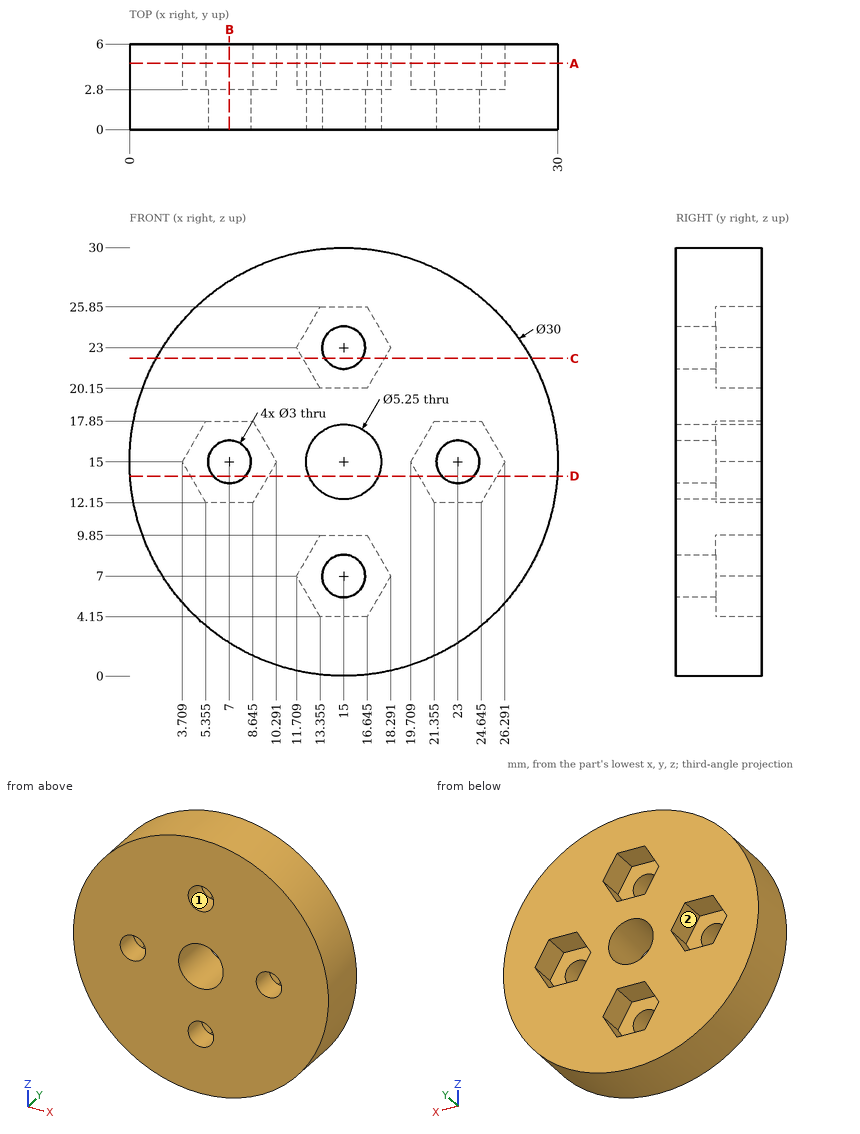
Source: three-view drawing plus pictorial views. Frame: mm from the lowest corner of the part. A direction names the side the tool comes from. Give positions to 0.01 mm unless a question says otherwise; leave off trailing zeros. Order: outer loops, then holes, each group sorted by start corner. A loop starts at its lowest first (then second) coordinate and runs counter-clockwise, first axis right, second up. Notation, with made-up numbers: M -30.5,26.25 L 25.5,26.25 A27 cw 25.5,47.25 Z; hole C 5,86 d5. An arc over 180 degrees is marked long. One line per question, with ' | ' between items. Start each with the question number.
1. First-contact query: pin 1 Ø1.6 at (x, y) = (7, 4) entering from -Z; pin 2 Ø5 at (x, z) = (15, 23) entering from +Y; pin 3 Ø2.5 at (x, y) = (23, 5) entering from -Z (1 decimal). Flat tips, straight axial feed; report the tip coordinate or a pass-through.
2. Material intervals for probe 1 along Z at (x, y) = (18, 4.4) (1 decimal); probe 2 along Z at (x, y) = (15.5, 2.85); probe 3 along X at (y, z) = (4, 14) (1 decimal), sorted ascending. Write a range as [from, to].
3. Access query for the marked faces 1 and 2. Directions: +Z, -Z, +X, -X, +Y, -Y. A direction counts if a zero-diameter tool reaches every point of the face in a straight line with its end or side. Return the directions, or none.
4. Section query C-C (z = 22.25). Return the cut outline in (x, y).
5. Section query A-A (y = 4.65). Count the separate pieces of the cut face and the enclosed holes in it.
6. Section query D-D (z = 14). Return the cut outline in (x, y), and give its area (3 significant figures).
7. Section query B-B (x = 7). Return the cut outline in (y, z), and give its area (3 significant figures).
Here are the results:
1) pin 1: z = 1.84 | pin 2: y = 2.8 | pin 3: z = 1.6
2) probe 1: [0.3, 6.5], [7.5, 22.5], [23.5, 29.7] | probe 2: [0.01, 4.15], [9.85, 12.42], [17.58, 20.15], [25.85, 29.99] | probe 3: [0, 4.3], [9.7, 12.6], [17.4, 20.3], [25.7, 30]
3) face 1: +Y, -Y | face 2: +Y
4) outline: M 1.87,0 L 13.7,0 L 13.7,2.8 L 12.14,2.8 L 12.14,6 L 1.87,6 Z; M 16.3,0 L 28.13,0 L 28.13,6 L 17.86,6 L 17.86,2.8 L 16.3,2.8 Z
5) separate pieces: 1 | enclosed holes: 5
6) outline: M 0.03,0 L 5.88,0 L 5.88,2.8 L 4.29,2.8 L 4.29,6 L 0.03,6 Z; M 8.12,0 L 12.57,0 L 12.57,6 L 9.71,6 L 9.71,2.8 L 8.12,2.8 Z; M 17.43,0 L 21.88,0 L 21.88,2.8 L 20.29,2.8 L 20.29,6 L 17.43,6 Z; M 24.12,0 L 29.97,0 L 29.97,6 L 25.71,6 L 25.71,2.8 L 24.12,2.8 Z | area: 103 mm²
7) outline: M 0,2.31 L 6,2.31 L 6,12.15 L 2.8,12.15 L 2.8,13.5 L 0,13.5 Z; M 0,16.5 L 2.8,16.5 L 2.8,17.85 L 6,17.85 L 6,27.69 L 0,27.69 Z | area: 126 mm²
